```python
from build123d import *

# Parameters (mm, degrees)
F1_DEPTH = 125.222
F2_R     = 5.08
F3_R     = 5.08
F4_R     = 11.212444
F5_DEPTH = 50.8


with BuildPart() as f1:
    # F0 (on Top) → F1 (new body)
    with BuildSketch(Plane.XY):
        Polygon((24.802748, 19.800747), (-28.966488, 33.822093), (-28.966488, -6.352786), (29.399224, -13.475696), align=None)
    extrude(amount=F1_DEPTH)

    # F2
    f2_edges = [f1.edges().sort_by_distance(p)[0] for p in [
        (27.100986, 3.162526, 125.222),
    ]]
    fillet(f2_edges, radius=F2_R)

    # F3
    f3_edges = [f1.edges().sort_by_distance(p)[0] for p in [
        (-28.966488, 13.734654, 125.222),
    ]]
    fillet(f3_edges, radius=F3_R)

    # F4 (on face) → F5 (join)
    with BuildSketch(Plane.XY.offset(125.222)):
        with Locations((5.875811, 12.488189)):
            Circle(F4_R)
    extrude(amount=F5_DEPTH)


solid = f1.part
```
Could you check a few things on this model? Use its own coordinates, in mm. A direction names the side the tool comes from. Give positions to 0.01 mm unless a question says otherwise; leave off trailing zeros. Write each loop counter-clockwise with the first axis right and the second up, starting at its lowest first coordinate (ties: lowest second). Pieces come first, ordered by that corner, then holes. Notation, with made-up numbers: (66, 40) - (102, 40) arc R19 ccw to (102, 63) - close; hole circle Ø5 at (24, 29). An arc over 180 degrees is marked (long way). One line per item, written item: value. Start each with the question number.
Item 1: I'm going to push flat-ended pins straight in: pin 1 (5 mm diameter, centred on x = 13, z = 74, fed in from -Y); pin 2 (6 mm diameter, centred on y = 8, z = 133, fed in from -X); pin 3 (6 mm diameter, centred on x = 18.5, z = 43.5, fed in from +Y). Where does each tip first touch, or does it pass through?
Item 2: Imagine slicing it at C-C, the plane y = 29.5. List the corners of the cut face in (x, z) for me.
Item 3: Which directions (+Z, -Z, +X, -X, +Y, -Y) give clear straight access to the entire face, cutting with the end or side of a thin tool? Please do faces 1 (the face through (25.49, 4.25, 123.69)), 2 (the face through (3.45, 1.54, 150.27)).
Item 4: Imagine slicing it at B-B, the plane z = 21. List the corners of the cut face in (x, y) for me.
Item 5: Imagine slicing it at D-D, the plane x = 8. List the corners of the cut face in (y, z) for me.
Item 6: Imagine slicing it at A-A, the plane x = -2. List the corners of the cut face in (y, z) for me.
Item 7: Please list where these lines run through material, in increasing order: line 1 (Z direction, x = 13, y = -8.5); line 2 (Z direction, x = 23, y = 16); line 3 (X direction, y = -5.5, z = 18). Write a range as from..to.
Geometry says:
1. pin 1: y = -11.78
1. pin 2: x = -5.24
1. pin 3: y = 22.23
2. outline: (-28.97, 0) - (-12.39, 0) - (-12.39, 125.22) - (-23.89, 125.22) arc R5.08 ccw to (-28.97, 120.14) - close
3. face 1: +Z, +X, +Y
3. face 2: +Z
4. outline: (-28.97, -6.35) - (29.4, -13.48) - (24.8, 19.8) - (-28.97, 33.82) - close
5. outline: (-10.86, 0) - (24.18, 0) - (24.18, 125.22) - (23.5, 125.22) - (23.5, 176.02) - (1.48, 176.02) - (1.48, 125.22) - (-10.86, 125.22) - close
6. outline: (-9.64, 0) - (26.79, 0) - (26.79, 125.22) - (20.47, 125.22) - (20.47, 176.02) - (4.51, 176.02) - (4.51, 125.22) - (-9.64, 125.22) - close
7. line 1: 0..125.22
7. line 2: 0..124.4
7. line 3: -28.97..28.3
